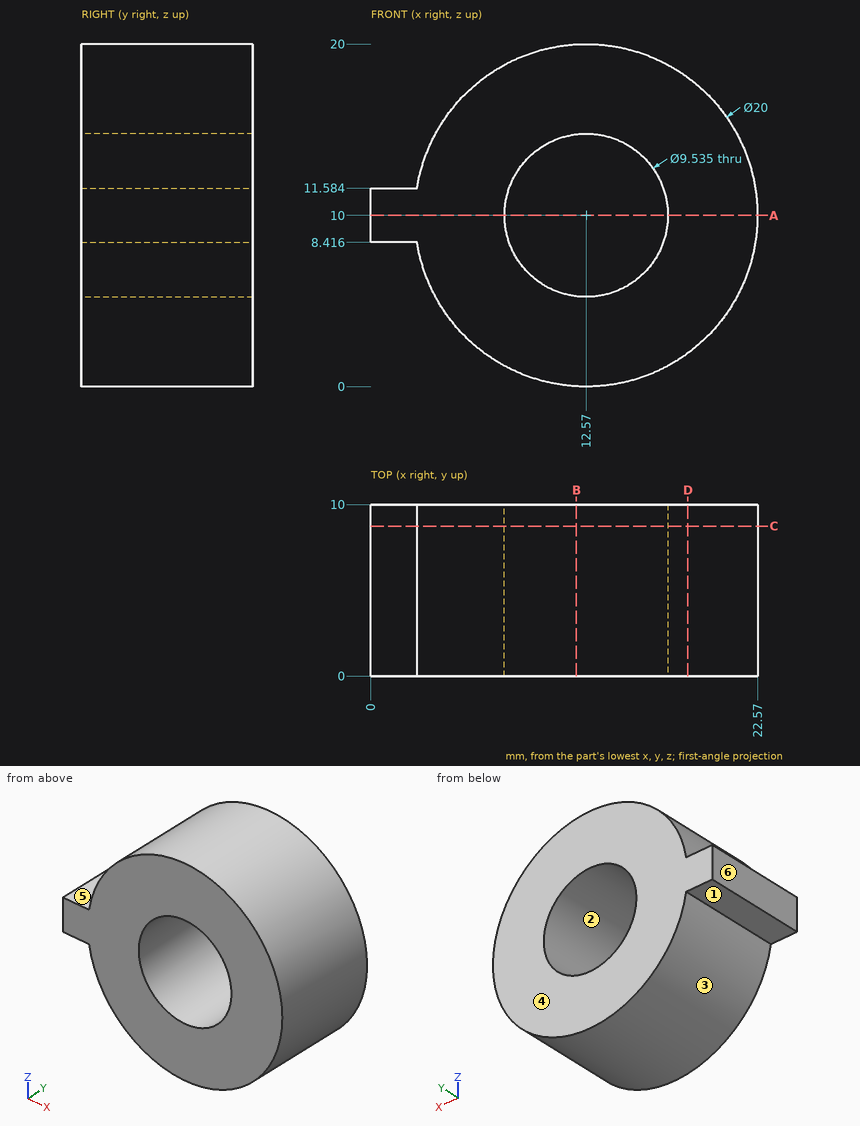
Print and shaded views of the part. All mm, measured from the part's lowest x, y and z. A direction names the side the tool comes from. Round coordinates to 2 decimals unless told otherwise and drop trailing zeros. Write each loop counter-clockwise with the first axis right and the second up, starting at its lowest first coordinate (ties: lowest second). Pieces come first, ordered by that corner, then holes. Notation, with made-up numbers: (77.25, 78.5) -> (93.25, 78.5) arc R15 cw to (93.25, 83.5) -> close; hole circle Ø7 at (88.5, -26). An arc over 180 degrees is marked (long way). Answer in a Markdown table with one row per item. Add a question column.
Item 1: Saw through at B-B, the plane x = 12. Write the cut outline in (y, z), then the cut area to 3 significant figures.
Item 2: Mould opens along Z. For the marked faces 1, 2, 3 and 4 say: pulls with the +Z half, pulls with the -Z half, needs draft (parallel to the pull), parting line crosses it, or undercut.
Item 3: Drop flat-ended pins along their axis: pin 1 Ø3 at (x, y) = (2, 5.5) entering from -Z; pin 2 Ø5.5 at (x, z) = (12.57, 10) entering from -Y; pin 3 Ø1 at (y, z) = (6, 7) entering from -X; pin 4 Ø2 at (x, y) = (1.5, 5.5) entering from +Z. Give the stop position or say it passes through.
Item 4: Saw through at A-A, the plane z = 10. Write the cut outline in (x, y), then the cut area to 3 significant figures.
Item 5: Saw through at D-D, the plane x = 18.5. Write the cut outline in (y, z), then the cut area to 3 significant figures.
Item 6: Which spindle directions (+Z, -Z, +X, -X, +Y, -Y) get a long thin tool onto all of the face, cutting with end or side? Do the marked faces 5 and 6. Say none if no direction does.
Item 7: Drill centre lines: line 1 (X direction, y = 1, z = 9.75); line 2 (Z direction, x = 2, y = 1.25); line 3 (X direction, y = 9, z = 13) (1 decimal). Where is each one in solid material? Low to high. Write a range as from..to.
Item 8: Saw through at C-C, the plane y = 8.75. Write the cut outline in (x, z) (1 decimal), then the cut area to 3 significant figures.
Findings below:
| question | item | result |
|---|---|---|
| 1 | outline | (0, 0.02) -> (10, 0.02) -> (10, 5.27) -> (0, 5.27) -> close; (0, 14.73) -> (10, 14.73) -> (10, 19.98) -> (0, 19.98) -> close |
| 1 | area | 105 mm^2 |
| 2 | face 1 | pulls with the -Z half |
| 2 | face 2 | undercut |
| 2 | face 3 | parting line crosses it |
| 2 | face 4 | needs draft |
| 3 | pin 1 | stops at z = 5.79 |
| 3 | pin 2 | passes through |
| 3 | pin 3 | stops at x = 2.89 |
| 3 | pin 4 | stops at z = 11.58 |
| 4 | outline | (0, 0) -> (7.8, 0) -> (7.8, 10) -> (0, 10) -> close; (17.34, 0) -> (22.57, 0) -> (22.57, 10) -> (17.34, 10) -> close |
| 4 | area | 130 mm^2 |
| 5 | outline | (0, 1.95) -> (10, 1.95) -> (10, 18.05) -> (0, 18.05) -> close |
| 5 | area | 161 mm^2 |
| 6 | face 5 | +Z, -X, +Y, -Y |
| 6 | face 6 | +Z, -Z, -X, +Y, -Y |
| 7 | line 1 | x = 0..7.81, 17.33..22.57 |
| 7 | line 2 | z = 8.42..11.58 |
| 7 | line 3 | x = 3..8.9, 16.3..22.1 |
| 8 | outline | (0, 8.4) -> (2.7, 8.4) arc R10 ccw (long way) to (2.7, 11.6) -> (0, 11.6) -> close; hole circle Ø9.5 at (12.6, 10) |
| 8 | area | 251 mm^2 |
